Verification items for the finished model (mm, model axes). A direction names the side the tool comes from. Round coordinates to 2 decimals unless told otherwise and drop trailing zeros. Order: outer loops, then holes, each group sorted by start corner. A loop starts at its lowest first (then second) coordinate and runs counter-clockwise, first axis right, second up. Notation, with made-up numbers: (34.25, 63.5) -> (64.25, 63.5) arc R29 ccw to (64.25, 101.5) -> close; hole circle Ø6 at (80, -31.75). An arc over 180 degrees is marked (long way). Return JSON: item names as keys, results as strings. Group by question number.
Item 1: Sectioned sample at A-A on z = 0. Record the cut outline in (x, y), plus the area to 3 significant figures.
Item 2: Sectioned sample at B-B on x = -5. Record the cut outline in (y, z), plus the area to 3 significant figures.
Item 3: Access from +Z, -Z, +X, -X, +Y, -Y to the whole of each face (thin tool, end or side, straight path). Record for faces 1 (the flat face through (3, 2, 0)), 2 (the flat face through (0, 1, -8)), 3 (the flat face through (0, 1, 7)).
Item 4: Sectioned sample at C-C on y = 1.8. Record the cut outline in (x, z).
Item 5: Sectioned sample at D-D on x = 1.5. Record the cut outline in (y, z), plus the area to 3 significant figures.
Item 6: Draft check along Z on faces 4 (the flat face through (1, 2, -5)), 5 (the flat face through (-3, 0, 0)), 6 (the cylindrical face through (-6.2, 1.5, 0.9)), 7 (the flat face through (2, 2, 5)). Enter one of: pulls with the +Z half, pulls with the -Z half, needs draft (parallel to the pull), parting line crosses it, or undercut.
Item 7: Scan lines: probe 1 along X at (y, z) = (1.2, 0); probe 2 along Z at (x, y) = (2, 0.65); probe 3 along Z at (x, y) = (-6, 2.8). Record each from-to range of solid material in increasing order. Write a range as from..to.
Item 8: Depth check by flat-ended pin: pin 1 Ø1 at (y, z) = (0.5, 4.5) entering from -X; pin 2 Ø1 at (x, y) = (-6.5, 0.5) entering from +Z; pin 3 Ø1.5 at (y, z) = (2.5, -7) entering from -X. Enter the tip coordinate at first touch or a pass-through.
Autodesk Inventor part; units mm, degrees
ref_plane "YZ Plane" through (0, 0, 0) normal (1, 0, 0) x (0, 1, 0)
ref_plane "XZ Plane" through (0, 0, 0) normal (0, 1, 0) x (-1, 0, 0)
ref_plane "XY Plane" through (0, 0, 0) normal (0, 0, 1) x (1, 0, 0)
sketch "Sketch1" plane through (0, 0, 0) normal (0, 1, 0) x (-1, 0, 0)
  circle A0 centre (0, 0) radius 10
  line L0 (0, -10) -> (0, 10)
  dimension "d0" = 20
extrude "Extrusion1" add sketch "Sketch1" along normal blind 3 contours A0 L0 picked at (2.6061, 2.0783)
sketch "Sketch2" plane through (0, 3, 0) normal (0, 1, 0) x (1, 0, 0)
  line L0 (0, 5) -> (3, 5)
  line L1 (3, 5) -> (3, -5)
  line L2 (3, -5) -> (0, -5)
  line L3 (0, -5) -> (0, 5)
  line L4 (0, -10) -> (0, 10)
  point P0 (0, 0)
  point P1 (3, 0)
  point P2 (0, 0)
  dimension "d3" = 3
  dimension "d4" = 10
extrude "Extrusion2" add sketch "Sketch2" against normal blind 3
sketch "Sketch3" plane through (0, 3, 0) normal (0, 1, 0) x (1, 0, 0)
  circle A0 centre (-5, 0) radius 1.5
  line L0 (0, -10) -> (0, -5)
  point P0 (0, 0)
  dimension "d7" = 3
  dimension "d8" = 5
extrude "Extrusion3" cut sketch "Sketch3" against normal blind 3
properties part number "Cradel holder"
Recorded:
{
 "1": {"outline": "(-10, 0) -> (-6.5, 0) -> (-6.5, 3) -> (-10, 3) -> close; (-3.5, 0) -> (3, 0) -> (3, 3) -> (-3.5, 3) -> close", "area": "30.0 mm²"},
 "2": {"outline": "(0, -8.66) -> (3, -8.66) -> (3, -1.5) -> (0, -1.5) -> close; (0, 1.5) -> (3, 1.5) -> (3, 8.66) -> (0, 8.66) -> close", "area": "43.0 mm²"},
 "3": {"face 1": "+Z, -Z, +X, +Y, -Y", "face 2": "-Z, +X, +Y, -Y", "face 3": "+Z, +X, +Y, -Y"},
 "4": {"outline": "(0, -10) -> (0, -5) -> (3, -5) -> (3, 5) -> (0, 5) -> (0, 10) arc R10 ccw to start; hole circle Ø3 at (-5, 0)"},
 "5": {"outline": "(0, -5) -> (3, -5) -> (3, 5) -> (0, 5) -> close", "area": "30.0 mm²"},
 "6": {"face 4": "pulls with the -Z half", "face 5": "needs draft", "face 6": "undercut", "face 7": "pulls with the +Z half"},
 "7": {"probe 1": "-10..-6.5, -3.5..3", "probe 2": "-5..5", "probe 3": "-8..-1.12, 1.12..8"},
 "8": {"pin 1": "x = -9.17", "pin 2": "z = 8", "pin 3": "x = -7.81"}
}
